from build123d import *

# Parameters (mm, degrees)
F0_W     = 25
F0_H     = 50
F1_DEPTH = 2
F2_DEPTH = 6
F3_R     = 3.99999


# Not quite as in the source:
# - a fillet or chamfer is up to 0.001 mm smaller than in the source, because OpenCascade refuses the exact size


with BuildPart() as f1:
    # F0 (on Top) → F1 (new body)
    with BuildSketch(Plane.XY):
        Polygon((8.9700092217, 2.9870720308), (8.9700092217, -2.0129279692), (48.3700092217, -2.0129279692), (48.3700092217, 2.9870720308), (49.2700092217, 52.9870720308), (49.2700092217, 57.9870720308), (8.0700092217, 57.9870720308), (8.1450092217, 52.9870720308), align=None)
        Polygon((41.1700092217, 2.9040758964), (41.1700092217, 2.9870720308), (16.1700092217, 2.9870720308), (13.9700092217, 2.9870720308), (13.9700092217, 52.9870720308), (16.1700092217, 52.9870720308), (41.1700092217, 52.9870720308), (43.3700092217, 52.9870720308), (43.3700092217, 2.9040758964), align=None, mode=Mode.SUBTRACT)
        Polygon((49.2700092217, 57.9870720308), (49.2700092217, 52.9870720308), (54.1950092217, 52.9870720308), (54.2700092217, 57.9870720308), align=None)
        Polygon((3.0700092217, 57.9870720308), (3.1450092217, 52.9870720308), (8.1450092217, 52.9870720308), (8.0700092217, 57.9870720308), align=None)
        Polygon((3.8950092217, 2.9870720308), (3.9700092217, -2.0129279692), (8.9700092217, -2.0129279692), (8.9700092217, 2.9870720308), align=None)
        Polygon((48.3700092217, 2.9870720308), (48.3700092217, -2.0129279692), (53.3700092217, -2.0129279692), (53.4438676036, 2.910964155), align=None)
        with Locations((28.6700092217, 27.9870720308)):
            Rectangle(F0_W, F0_H)
    extrude(amount=F1_DEPTH)

    # F0 (on Top) → F2 (join)
    with BuildSketch(Plane.XY):
        Polygon((3.8950092217, 2.9870720308), (3.9700092217, -2.0129279692), (8.9700092217, -2.0129279692), (8.9700092217, 2.9870720308), align=None)
        Polygon((48.3700092217, 2.9870720308), (48.3700092217, -2.0129279692), (53.3700092217, -2.0129279692), (53.4438676036, 2.910964155), align=None)
        Polygon((49.2700092217, 57.9870720308), (49.2700092217, 52.9870720308), (54.1950092217, 52.9870720308), (54.2700092217, 57.9870720308), align=None)
        Polygon((3.0700092217, 57.9870720308), (3.1450092217, 52.9870720308), (8.1450092217, 52.9870720308), (8.0700092217, 57.9870720308), align=None)
    extrude(amount=F2_DEPTH)

    # F3 (radius 4 in the source; OpenCascade refuses exactly that, so slightly less here)
    f3_edges = [f1.edges().sort_by_distance(p)[0] for p in [
        (8.970009, 0.487072, 6),
        (8.107509, 55.487072, 6),
        (49.270009, 55.487072, 6),
        (48.370009, 0.487072, 6),
    ]]
    fillet(f3_edges, radius=F3_R)


solid = f1.part
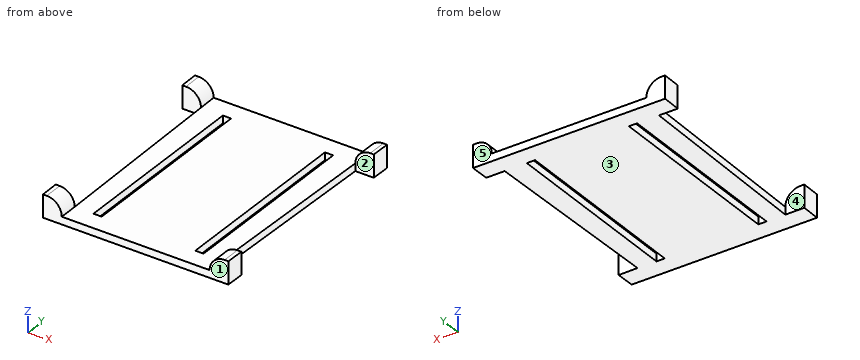
Source: CAD feature listing. Evaluate the final solid. Frame: model axes, mm. Face numbers are marked on the shaded views. A direction names the side the tool comes from. Round coordinates to 2 decimals unless told otherwise and drop trailing zeros. Order: outer loops, then holes, each group sorted by start corner. A loop starts at its lowest first (then second) coordinate and runs counter-clockwise, first axis right, second up. Notation, with made-up numbers: (9.25, 68.5) -> (27.25, 68.5) arc R22 cw to (27.25, 93.5) -> close; hole circle Ø7 at (-19.5, -38.75). An arc over 180 degrees is marked (long way). Answer as CSV lines item,"result".
Item 1: Line query: L1, parallel to X at y = 33, z = 0.5; L2, parallel to Y at x = 51.5, z = 2.75; L3, parallel to X at y = 50, z = 0.5. Output: solid intervals per line, ascending.
A:
L1,"8.47 to 13.97, 16.17 to 41.17, 43.37 to 48.91"
L2,"-2.01 to 2.94, 52.99 to 57.99"
L3,"8.19 to 13.97, 16.17 to 41.17, 43.37 to 49.22"
Item 2: Section B-B, the plane y = 10.5. Return loops of the section in (x, z), plus the area to 3 significant figures.
A:
outline,"(8.85, 0) -> (13.97, 0) -> (13.97, 2) -> (8.85, 2) -> close; (16.17, 0) -> (41.17, 0) -> (41.17, 2) -> (16.17, 2) -> close; (43.37, 0) -> (48.51, 0) -> (48.51, 2) -> (43.37, 2) -> close"
area,"70.5 mm²"
Item 3: Section C-C, the plane z = 5.25. Return loops of the section in (x, y) (3 decimals).
A:
outline,"(3.07, 57.987) -> (3.145, 52.987) -> (6.477, 52.987) -> (6.402, 57.987) -> close; (3.895, 2.987) -> (3.97, -2.013) -> (7.302, -2.013) -> (7.302, 2.987) -> close; (50.038, -2.013) -> (53.37, -2.013) -> (53.444, 2.911) -> (50.038, 2.962) -> close; (50.938, 52.987) -> (54.195, 52.987) -> (54.27, 57.987) -> (50.938, 57.987) -> close"
Item 4: Pin query (flat end, axial travel): pin 1 Ø12.5 at (x, y) = (26.5, 32.5) entering from +Z; pin 2 Ø1 at (y, z) = (38, 1) entering from +X; pin 3 Ø0.6 at (y, z) = (20.5, 1) entering from +X. Return the tip coordinate at first contact, or that it passes through.
A:
pin 1,"z = 2"
pin 2,"x = 49.01"
pin 3,"x = 48.69"
Item 5: Reachability of the marked faces 4 and 5 from +Z, -Z, +X, -X, +Y, -Y: full face, straight path, thin tool, end or side. Return the list, or none.
A:
face 4,"+Z, -Z, -X"
face 5,"+Z, -Z, +X, -X, +Y"
Item 6: Section D-D, the plane y = 42. Return loops of the section in (x, z).
A:
outline,"(8.33, 0) -> (13.97, 0) -> (13.97, 2) -> (8.33, 2) -> close; (16.17, 0) -> (41.17, 0) -> (41.17, 2) -> (16.17, 2) -> close; (43.37, 0) -> (49.07, 0) -> (49.07, 2) -> (43.37, 2) -> close"
Item 7: Pull-direction query (Y, two-part tool) for the marked faces 1, 2 and 3; classes: pulls with the +Y half, pulls with the -Y half, needs draft (parallel to the pull), parting line crosses it, or undercut.
A:
face 1,"pulls with the -Y half"
face 2,"undercut"
face 3,"needs draft"
Item 8: Section A-A, the plane z = 1. Return loops of the section in (x, y) (3 decimals), plus the area to 3 significant figures.
A:
outline,"(3.07, 57.987) -> (3.145, 52.987) -> (8.145, 52.987) -> (8.97, 2.987) -> (3.895, 2.987) -> (3.97, -2.013) -> (53.37, -2.013) -> (53.444, 2.911) -> (48.37, 2.987) -> (49.27, 52.987) -> (54.195, 52.987) -> (54.27, 57.987) -> close; hole (13.97, 2.987) -> (16.17, 2.987) -> (16.17, 52.987) -> (13.97, 52.987) -> close; hole (41.17, 2.904) -> (43.37, 2.904) -> (43.37, 52.987) -> (41.17, 52.987) -> close"
area,"2,300 mm²"
